Geometry: final body of the model. Coordinates: model frame, mm. Round coordinates to 2 decimals unless told otherwise and drop trailing zeros. Loops run counter-clockwise (first coordinate to the right, second up) from the corner with the lowest first, then second, coordinate; pieces in that order, holes last. Notation, with made-up numbers: (8, -7) - (40, -7) arc R35 cw to (40, 31) - close; hole circle Ø9 at (7.25, -3.75). An arc over 180 degrees is marked (long way). Use CSV: the item, a comma, the result in double quotes.
from build123d import *
from OCP.BRepFilletAPI import BRepFilletAPI_MakeChamfer

# Parameters (mm, degrees)
M3_CLEARANCE_HOLE1_D = 3.242
CHAMFER1_SIZE        = 0.378886114
CHAMFER1_SIZE2       = 0.21875
CHAMFER2_SIZE        = 2.507183156
CHAMFER2_SIZE2       = 2.507184174


with BuildPart() as part:
    # Sketch1 → Revolve1 (revolve)
    with BuildSketch(Plane(origin=(0, 0, 0), x_dir=(-1, 0, 0), z_dir=(0, 0, -1)), mode=Mode.PRIVATE) as revolve1_sk:
        Polygon((-3.2, 2.9), (-3.2, 0), (0, 0), (0, 2.9), (-1.6, 5.671281292), align=None)
    revolve(revolve1_sk.sketch.rotate(Axis((3.2, 0, 0), (-1, 0, 0)), 270), axis=Axis((3.2, 0, 0), (-1, 0, 0)))

    # M3 Clearance Hole1 (through all)
    with Locations(Plane.ZY):
        with Locations((0, 0)):
            Hole(M3_CLEARANCE_HOLE1_D / 2)

    # Chamfer1: one chamfer whose edges measure the first distance from different faces: ONE call of the kernel's chamfer builder (chamfer() names one face for all edges)
    chamfer1_edges_1 = [part.edges().sort_by_distance(p)[0] for p in [
        (0, 0, 1.621),
    ]]
    chamfer1_side_1 = [part.faces().sort_by_distance(p)[0] for p in [
        (0, 0, -2.817975613),
    ]]
    chamfer1_edges_2 = [part.edges().sort_by_distance(p)[0] for p in [
        (3.2, 0, 1.621),
    ]]
    chamfer1_side_2 = [part.faces().sort_by_distance(p)[0] for p in [
        (1.6, 0, 1.621),
    ]]
    chamfer1 = BRepFilletAPI_MakeChamfer(part.part.solid().wrapped)
    for e in chamfer1_edges_1:
        chamfer1.Add(CHAMFER1_SIZE, CHAMFER1_SIZE2, e.wrapped, chamfer1_side_1[0].wrapped)  # the first distance lies on this face
    for e in chamfer1_edges_2:
        chamfer1.Add(CHAMFER1_SIZE, CHAMFER1_SIZE2, e.wrapped, chamfer1_side_2[0].wrapped)  # the first distance lies on this face
    add(Compound.cast(chamfer1.Shape()), mode=Mode.REPLACE)

    # Chamfer2
    chamfer2_edges = [part.edges().sort_by_distance(p)[0] for p in [
        (1.6, 0, -5.671281292),
    ]]
    chamfer2_side = [part.faces().sort_by_distance(p)[0] for p in [
        (2.4, 0, -4.285640646),
    ]]
    chamfer(chamfer2_edges, length=CHAMFER2_SIZE, length2=CHAMFER2_SIZE2, reference=chamfer2_side[0])


solid = part.part
Item 1: Section A-A on x = 2.95. Return the cut outline in (y, z).
Final values:
outline,"circle Ø6.67 at (0, 0); hole circle Ø3.39 at (0, 0)"
Item 2: Mould query, pull axis Y, two halves, no side actions, for faces 1 (the flat face through (3.2, -2, 0)), 2 (the cylindrical face through (1.538, -1.438, -0.748)). Classes: released by +Y, released by -Y, zero draft, split by the parting line, or undercut.
Final values:
face 1,"zero draft"
face 2,"undercut"
Item 3: Pin query (flat end, axial travel): P1, Ø1.5, axis at x = 3, y = 2.5, coming from the -Z side; P2, Ø3, axis at y = 0, z = 0, coming from the +X side. Return the tip coordinate at first contact, or that it passes through.
Final values:
P1,"stops at z = -3.02"
P2,"passes through"
Item 4: Material intervals for line 1 (Y direction, x = 2.15, z = 0); line 2 (Y direction, x = 2.05, z = -0.75); line 3 (Z direction, x = 2.4, y = 1.25), sorted ascending.
Final values:
line 1,"y = -3.5 to -1.62, 1.62 to 3.5"
line 2,"y = -3.42 to -1.44, 1.44 to 3.42"
line 3,"z = -3.27 to -1.03, 1.03 to 3.27"
